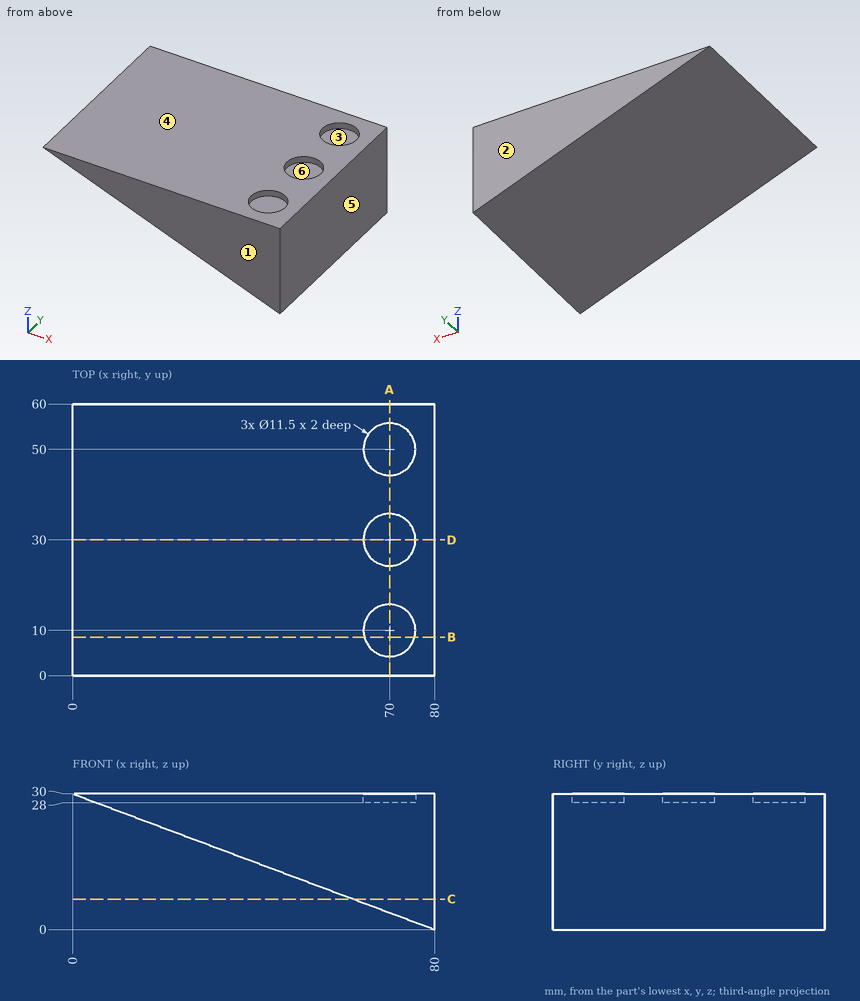
Study the drawing (mm; zero at the part's minimum x, y, z) and answer. A direction names the side the tool comes from. Give positions to 0.01 mm unless a question says otherwise; leave off trailing zeros. Write each loop counter-clockwise with the first axis right and the second up, starting at its lowest first coordinate (ties: lowest second). Pieces come first, ordered by that corner, then holes. Notation, with made-up numbers: (-21.5, -37) -> (30.5, -37) arc R15 cw to (30.5, -14) -> close; hole circle Ø9 at (-33, -21). An arc over 180 degrees is marked (long way). Answer in a Markdown table with one row per item.
1) Determine the mould class of the marked faces 1, 2, 3 and 4 for opening direction Y: released by +Y, released by -Y, zero draft, split by the parting line, or undercut.
Results list:
| item | result |
|---|---|
| face 1 | released by -Y |
| face 2 | released by +Y |
| face 3 | undercut |
| face 4 | zero draft |
2) Each of these flat-tipped pins is pushed along its axis until it touches: pin 1 Ø7 at (x, y) = (70, 30) entering from -Z; pin 2 Ø9 at (x, y) = (70, 10) entering from -Z; pin 3 Ø7 at (x, y) = (70, 50) entering from +Z. Where does it stop, or does it pass through?
Results list:
| item | result |
|---|---|
| pin 1 | z = 2.44 |
| pin 2 | z = 2.06 |
| pin 3 | z = 28 |
3) Straight lines are drawn through the part: line 1 (Y direction, x = 70, z = 29.55); line 2 (Z direction, x = 67, y = 11.5) (3 decimals); line 3 (Z direction, x = 9, y = 9) (3 decimals). For each, find the intervals that lie inside material, in ascending order. Write a range as [from, to].
Results list:
| item | result |
|---|---|
| line 1 | [0, 4.25], [15.75, 24.25], [35.75, 44.25], [55.75, 60] |
| line 2 | [4.875, 28] |
| line 3 | [26.625, 30] |
4) Section D-D on y = 30 is taken. Give the vertices of the cut face in (x, z), plus the area to 3 significant figures.
Results list:
| item | result |
|---|---|
| outline | (0, 30) -> (80, 0) -> (80, 30) -> (75.75, 30) -> (75.75, 28) -> (64.25, 28) -> (64.25, 30) -> close |
| area | 1,180 mm^2 |
5) Section B-B on y = 8.5 is taken. Give the vertices of the cut face in (x, z), plus the area to 3 significant figures.
Results list:
| item | result |
|---|---|
| outline | (0, 30) -> (80, 0) -> (80, 30) -> (75.55, 30) -> (75.55, 28) -> (64.45, 28) -> (64.45, 30) -> close |
| area | 1,180 mm^2 |
6) Section C-C on z = 6.75 is taken. Give the vertices of the cut face in (x, y), plus the area to 3 significant figures.
Results list:
| item | result |
|---|---|
| outline | (62, 0) -> (80, 0) -> (80, 60) -> (62, 60) -> close |
| area | 1,080 mm^2 |
7) Section A-A on x = 70 is taken. Give the vertices of the cut face in (y, z).
Results list:
| item | result |
|---|---|
| outline | (0, 3.75) -> (60, 3.75) -> (60, 30) -> (55.75, 30) -> (55.75, 28) -> (44.25, 28) -> (44.25, 30) -> (35.75, 30) -> (35.75, 28) -> (24.25, 28) -> (24.25, 30) -> (15.75, 30) -> (15.75, 28) -> (4.25, 28) -> (4.25, 30) -> (0, 30) -> close |
8) A tool of negligible diameter and unlimited length cuts with its end or side. For the marked faces 5 and 6, from which of +Z, -Z, +X, -X, +Y, -Y can it reach the whole face along a straight path? Write none if from no direction.
Results list:
| item | result |
|---|---|
| face 5 | +Z, -Z, +X, +Y, -Y |
| face 6 | +Z |
